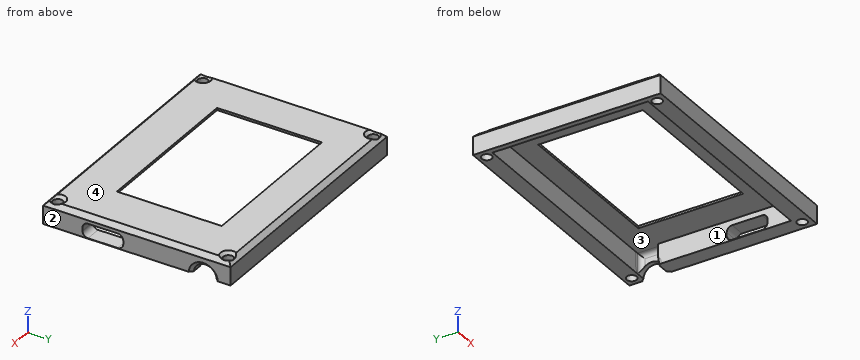
from build123d import *

# Parameters (mm, degrees)
SKETCH1_W                                       = 54.65
SKETCH1_H                                       = 41.15
BOSS_EXTRUDE1_DEPTH                             = 5
SKETCH2_W                                       = 35
SKETCH2_H                                       = 23
CUT_EXTRUDE1_DEPTH                              = 1.5
SKETCH3_W                                       = 47.65
SKETCH3_H                                       = 34.15
CUT_EXTRUDE2_DEPTH                              = 4.5
SKETCH4_R                                       = 2.5
CUT_EXTRUDE3_DEPTH                              = 4
CHAMFER1_SIZE                                   = 0.7
CSK_FOR_M3_FLAT_HEAD_MACHINE_SCREW1_D           = 2.2
CSK_FOR_M3_FLAT_HEAD_MACHINE_SCREW1_DEPTH       = 6
CSK_FOR_M3_FLAT_HEAD_MACHINE_SCREW1_CSINK_D     = 3.5
CSK_FOR_M3_FLAT_HEAD_MACHINE_SCREW1_CSINK_ANGLE = 90
CSK_FOR_M3_FLAT_HEAD_MACHINE_SCREW1_TIP         = 0.660946681
CHAMFER2_SIZE                                   = 1
FILLET3_R                                       = 0.75
CUT_EXTRUDE4_REACH                              = 70.593
SKETCH7_W                                       = 3.26
SKETCH7_H                                       = 8.94
FILLET4_R                                       = 1.2
BOSS_EXTRUDE2_DEPTH                             = 10
BOSS_EXTRUDE2_DEPTH_BACK                        = 0.1
SKETCH8_W                                       = 3.5
SKETCH8_H                                       = 8.94
FILLET5_R                                       = 1.2
CUT_EXTRUDE5_DEPTH                              = 65.35505355
CUT_EXTRUDE5_DEPTH_BACK                         = 65.35505355
SKETCH9_W                                       = 3.5
SKETCH9_H                                       = 10
SKETCH10_W                                      = 4.5
SKETCH10_H                                      = 34.15
CUT_EXTRUDE6_DEPTH                              = 2.3
CUT_EXTRUDE7_START                              = -4.5
SKETCH11_W                                      = 3.064355189
SKETCH11_H                                      = 4.983974318
CUT_EXTRUDE7_DEPTH                              = 4.5
FILLET6_R                                       = 1


with BuildPart() as part:
    # Sketch1 → Boss-Extrude1 (new body)
    with BuildSketch(Plane.XY):
        with Locations((27.325, 20.575)):
            Rectangle(SKETCH1_W, SKETCH1_H)
    extrude(amount=BOSS_EXTRUDE1_DEPTH)

    # Sketch2 → Cut-Extrude1 (cut)
    with BuildSketch(Plane.XY.offset(5)):
        with Locations((27.01, 21.34)):
            Rectangle(SKETCH2_W, SKETCH2_H)
    extrude(amount=-CUT_EXTRUDE1_DEPTH, mode=Mode.SUBTRACT)

    # Sketch3 → Cut-Extrude2 (cut)
    with BuildSketch(Plane(origin=(0, 0, 0), x_dir=(-1, 0, 0), z_dir=(0, 0, -1))):
        with Locations((-27.325, 20.575)):
            Rectangle(SKETCH3_W, SKETCH3_H)
    extrude(amount=-CUT_EXTRUDE2_DEPTH, mode=Mode.SUBTRACT)

    # Sketch4 → Cut-Extrude3 (cut)
    with BuildSketch(Plane(origin=(54.65, 0, 0), x_dir=(0, 0, -1), z_dir=(1, 0, 0))):
        with Locations((0.2, 35.15)):
            Circle(SKETCH4_R)
    extrude(amount=-CUT_EXTRUDE3_DEPTH, mode=Mode.SUBTRACT)

    # Chamfer1
    chamfer1_edges = [part.edges().sort_by_distance(p)[0] for p in [
        (54.65, 35.15, 2.3),
    ]]
    chamfer(chamfer1_edges, length=CHAMFER1_SIZE)

    # CSK for M3 Flat Head Machine Screw1
    with Locations(Plane.XY.offset(5)):
        with Locations((52.65, 2), (2, 39.4), (52.65, 39.4), (2, 2)):
            CounterSinkHole(CSK_FOR_M3_FLAT_HEAD_MACHINE_SCREW1_D / 2, CSK_FOR_M3_FLAT_HEAD_MACHINE_SCREW1_CSINK_D / 2, depth=CSK_FOR_M3_FLAT_HEAD_MACHINE_SCREW1_DEPTH, counter_sink_angle=CSK_FOR_M3_FLAT_HEAD_MACHINE_SCREW1_CSINK_ANGLE)
            with Locations((0, 0, -(CSK_FOR_M3_FLAT_HEAD_MACHINE_SCREW1_DEPTH + CSK_FOR_M3_FLAT_HEAD_MACHINE_SCREW1_TIP / 2))):  # 118° drill point
                Cone(0, CSK_FOR_M3_FLAT_HEAD_MACHINE_SCREW1_D / 2, CSK_FOR_M3_FLAT_HEAD_MACHINE_SCREW1_TIP, mode=Mode.SUBTRACT)

    # Chamfer2
    # the kernel refuses this chamfer: 1 mm, written as the material it takes off along each edge
    with BuildSketch(Plane(origin=(-0.571682988, 41.15, 5), x_dir=(0, -0.9996219169112968, 0.027495876610586414), z_dir=(1, 0, 0))) as chamfer2_piece_1:
        Polygon((CHAMFER2_SIZE * 0.999621916911, CHAMFER2_SIZE * 0.0274958766106), (-CHAMFER2_SIZE * 0.0274958766106, CHAMFER2_SIZE * 0.999621916911), (0, 0), align=None)
    extrude(amount=55.793365976, mode=Mode.SUBTRACT)
    with BuildSketch(Plane(origin=(54.65, 43.721682988, 5), x_dir=(0.02749587661058907, 0, -0.9996219169112965), z_dir=(0, -1, 0)), Plane(origin=(0, -2.571682988, 5), x_dir=(-0.027495876610586365, 0, -0.9996219169112968), z_dir=(0, 1, 0))) as chamfer2_piece_2:
        Polygon((CHAMFER2_SIZE * 0.999621916911, -CHAMFER2_SIZE * 0.0274958766106), (-CHAMFER2_SIZE * 0.0274958766106, -CHAMFER2_SIZE * 0.999621916911), (0, 0), align=None)
    extrude(amount=46.293365976, mode=Mode.SUBTRACT)
    with BuildSketch(Plane(origin=(57.221682988, 0, 5), x_dir=(0, -0.027495876610586365, -0.9996219169112968), z_dir=(-1, 0, 0))) as chamfer2_piece_3:
        Polygon((CHAMFER2_SIZE * 0.999621916911, -CHAMFER2_SIZE * 0.0274958766106), (-CHAMFER2_SIZE * 0.0274958766106, -CHAMFER2_SIZE * 0.999621916911), (0, 0), align=None)
    extrude(amount=59.793365976, mode=Mode.SUBTRACT)

    # Fillet3
    fillet3_edges = [part.edges().sort_by_distance(p)[0] for p in [
        (51.15, 35.15, 2.3),
    ]]
    fillet(fillet3_edges, radius=FILLET3_R)

    # Sketch7 → Cut-Extrude4 (cut, up to next)
    with BuildSketch(Plane(origin=(54.65, 0, 0), x_dir=(0, 0, -1), z_dir=(1, 0, 0)), mode=Mode.PRIVATE) as cut_extrude4_sk1:
        with Locations((-1.63, 13.14)):
            Rectangle(SKETCH7_W, SKETCH7_H)
    cut_extrude4_tool1 = extrude(cut_extrude4_sk1.sketch, amount=-CUT_EXTRUDE4_REACH, mode=Mode.PRIVATE) & part.part
    add(cut_extrude4_tool1.solids().sort_by_distance((54.65, 13.14, 1.63))[0], mode=Mode.SUBTRACT)

    # Fillet4
    fillet4_edges = [part.edges().sort_by_distance(p)[0] for p in [
        (52.9, 8.67, 3.26),
        (52.9, 17.61, 3.26),
    ]]
    fillet(fillet4_edges, radius=FILLET4_R)

    # Sketch8 → Boss-Extrude2 (add, two sides: drawn at the far end of the back side and taken through both)
    with BuildSketch(Plane(origin=(0, 0, 0), x_dir=(-1, 0, 0), z_dir=(0, 0, -1)).offset(-BOSS_EXTRUDE2_DEPTH_BACK)):
        with Locations((-52.9, 13.14)):
            Rectangle(SKETCH8_W, SKETCH8_H)
    extrude(amount=BOSS_EXTRUDE2_DEPTH + BOSS_EXTRUDE2_DEPTH_BACK)

    # Fillet5
    fillet5_edges = [part.edges().sort_by_distance(p)[0] for p in [
        (52.9, 17.61, 0.1),
        (52.9, 8.67, 0.1),
    ]]
    fillet(fillet5_edges, radius=FILLET5_R)

    # Sketch9 → Cut-Extrude5 (cut, two sides: drawn at the far end of the back side and taken through both)
    with BuildSketch(Plane.XZ.offset(-8.67).offset(-CUT_EXTRUDE5_DEPTH_BACK)):
        with Locations((52.9, -5)):
            Rectangle(SKETCH9_W, SKETCH9_H)
    extrude(amount=CUT_EXTRUDE5_DEPTH + CUT_EXTRUDE5_DEPTH_BACK, mode=Mode.SUBTRACT)

    # Sketch10 → Cut-Extrude6 (cut)
    with BuildSketch(Plane(origin=(3.5, 0, 0), x_dir=(0, 0, -1), z_dir=(1, 0, 0))):
        with Locations((-2.25, 20.575)):
            Rectangle(SKETCH10_W, SKETCH10_H)
    extrude(amount=-CUT_EXTRUDE6_DEPTH, mode=Mode.SUBTRACT)

    # Sketch11 → Cut-Extrude7 (cut)
    with BuildSketch(Plane(origin=(0, 0, 0), x_dir=(-1, 0, 0), z_dir=(0, 0, -1)).offset(CUT_EXTRUDE7_START)):
        with Locations((-51.392822405, 35.15)):
            Rectangle(SKETCH11_W, SKETCH11_H)
    extrude(amount=CUT_EXTRUDE7_DEPTH, mode=Mode.SUBTRACT)

    # Fillet6
    # the kernel refuses this fillet: 1 mm, written as the material it adds along each edge
    with BuildSketch(Plane(origin=(52.925, 32.658012841, 7), x_dir=(-1, 0, 0), z_dir=(0, 0, -1))) as fillet6_piece_1_section:
        with BuildLine():
            CenterArc((FILLET6_R, FILLET6_R), FILLET6_R, 180, 90)
            Line((0, FILLET6_R), (0, 0))
            Line((0, 0), (FILLET6_R, 0))
        make_face()
    fillet6_piece_1 = extrude(amount=7, mode=Mode.PRIVATE)
    fillet6_piece_1 = fillet6_piece_1 - Plane(origin=(52.688942882, 35.15, -0.2), x_dir=(0, 0, -1), z_dir=(1, 0, 0)) * Cylinder(2.5, 18, mode=Mode.PRIVATE)
    fillet6_piece_1 = split(fillet6_piece_1, bisect_by=Plane(origin=(52.688942882, 32.861757349, 5), z_dir=(0, 0, -1)), keep=Keep.TOP, mode=Mode.PRIVATE)
    add(fillet6_piece_1)
    with BuildSketch(Plane(origin=(52.925, 30.158012841, 4.5), x_dir=(-1, 0, 0), z_dir=(0, 1, 0))) as fillet6_piece_2:
        with BuildLine():
            CenterArc((FILLET6_R, -FILLET6_R), FILLET6_R, 90, 90)
            Line((0, -FILLET6_R), (0, 0))
            Line((0, 0), (FILLET6_R, 0))
        make_face()
    extrude(amount=7.483974318)
    with BuildSketch(Plane(origin=(52.925, 37.641987159, 7), x_dir=(0, -1, 0), z_dir=(0, 0, -1))) as fillet6_piece_3_section:
        with BuildLine():
            CenterArc((FILLET6_R, FILLET6_R), FILLET6_R, 180, 90)
            Line((0, FILLET6_R), (0, 0))
            Line((0, 0), (FILLET6_R, 0))
        make_face()
    fillet6_piece_3 = extrude(amount=7, mode=Mode.PRIVATE)
    fillet6_piece_3 = fillet6_piece_3 - Plane(origin=(52.688929228, 35.15, -0.2), x_dir=(0, 0, -1), z_dir=(1, 0, 0)) * Cylinder(2.5, 18, mode=Mode.PRIVATE)
    fillet6_piece_3 = split(fillet6_piece_3, bisect_by=Plane(origin=(52.688929228, 37.438232823, 5), z_dir=(0, 0, -1)), keep=Keep.TOP, mode=Mode.PRIVATE)
    add(fillet6_piece_3)


solid = part.part
Verification items for the finished model (mm, model axes). Face numbers are marked on the shaded views. A direction names the side the tool comes from. Round coordinates to 2 decimals unless told otherwise and drop trailing zeros. Order: outer loops, then holes, each group sorted by start corner. A loop starts at its lowest first (then second) coordinate and runs counter-clockwise, first axis right, second up.
1. Section check B-B on x = 41. Record the cut outline in (y, z), then the cut area to 3 significant figures.
Final values:
outline: (0, 0) - (3.5, 0) - (3.5, 4.5) - (9.84, 4.5) - (9.84, 5) - (1, 5) - (0, 4) - close; (32.84, 4.5) - (37.65, 4.5) - (37.65, 0) - (41.15, 0) - (41.15, 4) - (40.15, 5) - (32.84, 5) - close
area: 39.6 mm2
2. Section check A-A on y = 12. Record the cut outline in (x, z), then the cut area to 3 significant figures.
Final values:
outline: (0, 0) - (1.2, 0) - (1.2, 4.5) - (9.51, 4.5) - (9.51, 5) - (1, 5) - (0, 4) - close; (44.51, 4.5) - (51.15, 4.5) - (51.15, 3.26) - (54.65, 3.26) - (54.65, 4) - (53.65, 5) - (44.51, 5) - close; (51.15, 0) - (54.65, 0) - (54.65, 0.1) - (51.15, 0.1) - close
area: 18.9 mm2
3. Thickness scan on L1, parallel to Y at x = 2, z = 1.2; L2, parallel to X at y = 2, z = 1.2; L3, parallel to Y at x = 40, z = 1.05. Record the ranges inside material, lowest first.
Final values:
L1: y = 0 to 0.9, 3.1 to 3.5, 37.65 to 38.3, 40.5 to 41.15
L2: x = 0 to 0.9, 3.1 to 51.55, 53.75 to 54.65
L3: y = 0 to 3.5, 37.65 to 41.15
4. Access from +Z, -Z, +X, -X, +Y, -Y to the whole of each face (thin tool, end or side, straight path). Record for the marked faces 1 and 2.
Final values:
face 1: -Z
face 2: +Z, -Z, +X, +Y, -Y
5. Section check D-D on y = 35.15. Record the cut outline in (x, z) (3 decimals), then the cut area to 3 significant figures.
Final values:
outline: (0, 0) - (1.2, 0) - (1.2, 4.5) - (51.925, 4.5) arc R1 cw to (52.925, 3.5) - (52.925, 2.3) - (53.95, 2.3) - (54.65, 3) - (54.65, 4) - (53.65, 5) - (1, 5) - (0, 4) - close
area: 35.5 mm2
6. Release check for a two-part mould opening along Y. For the marked faces 3 and 4 record: +Y half, -Y half, draft (parallel to the pull), parting line (faces both ways), or undercut.
Final values:
face 3: undercut
face 4: draft
7. Go/stop test with flat-tipped pins: P1, Ø2.5, axis at x = 2, y = 39.4, coming from the +Z side; P2, Ø0.6, axis at y = 20.5, z = 4.5, coming from the -X side. Record where each tip stops, or that it passes through.
Final values:
P1: stops at z = 4.5
P2: stops at x = 0.2
8. Section check C-C on x = 2. Record the cut outline in (y, z) (3 decimals), then the cut area to 3 significant figures.
Final values:
outline: (0, 0) - (0.9, 0) - (0.9, 4.35) - (0.625, 4.625) - (0, 4) - close; (3.1, 0) - (3.5, 0) - (3.5, 4.5) - (37.65, 4.5) - (37.65, 0) - (38.3, 0) - (38.3, 4.35) - (37.65, 5) - (3.75, 5) - (3.1, 4.35) - close; (40.5, 0) - (41.15, 0) - (41.15, 4) - (40.65, 4.5) - (40.5, 4.35) - close
area: 28.6 mm2
